For this review, take the finished solid that the model builds, in its own axes (mm). Round coordinates to 2 decimals unless told otherwise and drop trailing zeros. Write each loop counter-clockwise with the first axis right and the second up, starting at its lowest first coordinate (ties: lowest second). Pieces come first, ordered by that corner, then holes.
from build123d import *

# Parameters (mm, degrees)
BASE_DEPTH                     = 5.999988
MOUNTING_HOLES_D               = 4.4958
MOUNTING_HOLES_DEPTH           = 5.9944
SKETCH5_W                      = 6
SKETCH5_H                      = 12.7
F_4_BAR_MOUNT_DEPTH            = 131.351874194
SKETCH8_R                      = 2.2479
LIMIT_SWITCH_MOUNT_HOLES_DEPTH = 131.351874194
LIM_SW_CIRC_PATTERN_COUNT      = 2
SKETCH9_W                      = 25.4
SKETCH9_H                      = 63.5
SKETCH9_W_2                    = 47.975
WIRE_HOLES_DEPTH               = 131.351874194
FILLET1_R                      = 3.81


with BuildPart() as part:
    # Sketch1 → Base (new body)
    with BuildSketch(Plane(origin=(0, 0, 0), x_dir=(1, 0, 0), z_dir=(0, 1, 0))):
        Polygon((-38.138713756, 92.075), (-92.075, 38.138713756), (-92.075, -38.138713756), (-38.138713756, -92.075), (38.138713756, -92.075), (92.075, -38.138713756), (92.075, 38.138713756), (38.138713756, 92.075), align=None)
    extrude(amount=BASE_DEPTH)

    # Mounting holes
    with Locations(Plane(origin=(0, 5.999988, 0), x_dir=(1, 0, 0), z_dir=(0, 1, 0))):
        with Locations((-35.508457634, 85.725), (35.508457634, 85.725), (85.725, 35.508457634), (85.725, -35.508457634), (35.508457634, -85.725), (-35.508457634, -85.725), (-85.725, -35.508457634), (-85.725, 35.508457634)):
            Hole(MOUNTING_HOLES_D / 2, depth=MOUNTING_HOLES_DEPTH)

    # Sketch5 → 4-bar mount (cut, through all)
    with BuildSketch(Plane(origin=(0, 5.999988, 0), x_dir=(1, 0, 0), z_dir=(0, 1, 0))):
        with Locations((-22.05, 25.4)):
            Rectangle(SKETCH5_W, SKETCH5_H)
        with Locations((-22.05, -25.4)):
            Rectangle(SKETCH5_W, SKETCH5_H)
        with Locations((-22.05, 0)):
            Rectangle(SKETCH5_W, SKETCH5_H)
        with Locations((22.05, 0)):
            Rectangle(SKETCH5_W, SKETCH5_H)
        with Locations((22.05, -25.4)):
            Rectangle(SKETCH5_W, SKETCH5_H)
        with Locations((22.05, 25.4)):
            Rectangle(SKETCH5_W, SKETCH5_H)
    extrude(amount=-F_4_BAR_MOUNT_DEPTH, mode=Mode.SUBTRACT)

    # Sketch8 → limit switch mount holes (cut, through all)
    with BuildSketch(Plane(origin=(0, 5.999988, 0), x_dir=(1, 0, 0), z_dir=(0, 1, 0))):
        with Locations(Location((-35.508457634, 66.675, 0), (0, 0, 270))):
            Circle(SKETCH8_R)
        with Locations(Location((-23.67230509, 66.675, 0), (0, 0, 270))):
            Circle(SKETCH8_R)
        with Locations(Location((-11.836152545, 66.675, 0), (0, 0, 270))):
            Circle(SKETCH8_R)
        with Locations(Location((0, 66.675, 0), (0, 0, 270))):
            Circle(SKETCH8_R)
        with Locations(Location((11.836152545, 66.675, 0), (0, 0, 270))):
            Circle(SKETCH8_R)
        with Locations(Location((23.67230509, 66.675, 0), (0, 0, 270))):
            Circle(SKETCH8_R)
        with Locations(Location((35.508457634, 66.675, 0), (0, 0, 270))):
            Circle(SKETCH8_R)
    limit_switch_mount_holes = extrude(amount=-LIMIT_SWITCH_MOUNT_HOLES_DEPTH, mode=Mode.SUBTRACT)

    # lim sw circ pattern: limit switch mount holes ×2 about axis
    lim_sw_circ_pattern_axis = Axis((0, 0, 0), (0, 1, 0))
    for i in range(1, LIM_SW_CIRC_PATTERN_COUNT):
        add(limit_switch_mount_holes.rotate(lim_sw_circ_pattern_axis, i * 360 / LIM_SW_CIRC_PATTERN_COUNT), mode=Mode.SUBTRACT)

    # Sketch9 → Wire holes (cut, through all)
    with BuildSketch(Plane(origin=(0, 5.999988, 0), x_dir=(1, 0, 0), z_dir=(0, 1, 0))):
        Rectangle(SKETCH9_W, SKETCH9_H)
        with Locations((-55.3875, 0)):
            Rectangle(SKETCH9_W_2, SKETCH9_H)
        with Locations((55.3875, 0)):
            Rectangle(SKETCH9_W_2, SKETCH9_H)
        Polygon((-74.153201513, 38.1), (74.153201513, 38.1), (51.928201513, 60.325), (-51.928201513, 60.325), align=None)
        Polygon((-74.153201513, -38.1), (74.153201513, -38.1), (51.928201513, -60.325), (-51.928201513, -60.325), align=None)
    extrude(amount=-WIRE_HOLES_DEPTH, mode=Mode.SUBTRACT)

    # Fillet1
    fillet1_edges = [part.edges().sort_by_distance(p)[0] for p in [
        (-12.7, 2.999994, 31.75),
        (-12.7, 2.999994, -31.75),
        (12.7, 2.999994, -31.75),
        (12.7, 2.999994, 31.75),
        (-79.375, 2.999994, 31.75),
        (-79.375, 2.999994, -31.75),
        (-31.4, 2.999994, -31.75),
        (-31.4, 2.999994, 31.75),
        (31.4, 2.999994, 31.75),
        (31.4, 2.999994, -31.75),
        (79.375, 2.999994, -31.75),
        (79.375, 2.999994, 31.75),
        (-74.153201513, 2.999994, -38.1),
        (-51.928201513, 2.999994, -60.325),
        (51.928201513, 2.999994, -60.325),
        (74.153201513, 2.999994, -38.1),
        (-51.928201513, 2.999994, 60.325),
        (-74.153201513, 2.999994, 38.1),
        (74.153201513, 2.999994, 38.1),
        (51.928201513, 2.999994, 60.325),
    ]]
    fillet(fillet1_edges, radius=FILLET1_R)


solid = part.part
(1) We need section B-B, the plane x = 0. Give the boundary of the cut face in (y, z) (3 decimals), and give its area (3 significant figures).
Geometry check:
outline: (0, -92.075) - (6, -92.075) - (6, -68.923) - (0, -68.923) - close; (0, -64.427) - (6, -64.427) - (6, -60.325) - (0, -60.325) - close; (0, -38.1) - (6, -38.1) - (6, -31.75) - (0, -31.75) - close; (0, 31.75) - (6, 31.75) - (6, 38.1) - (0, 38.1) - close; (0, 60.325) - (6, 60.325) - (6, 64.427) - (0, 64.427) - close; (0, 68.923) - (6, 68.923) - (6, 92.075) - (0, 92.075) - close
area: 403 mm2
(2) We need section C-C, the plane z = -52.5. Give the boundary of the cut face in (x, y).
Geometry check:
outline: (-77.71, 0) - (-59.75, 0) - (-59.75, 6) - (-77.71, 6) - close; (59.75, 0) - (77.71, 0) - (77.71, 6) - (59.75, 6) - close
(3) We need section D-D, the plane x = 73. Give the boundary of the cut face in (y, z), and give its area (3 significant figures).
Geometry check:
outline: (0, -57.21) - (6, -57.21) - (6, -31.75) - (0, -31.75) - close; (0, 31.75) - (6, 31.75) - (6, 57.21) - (0, 57.21) - close
area: 306 mm2
(4) We need section A-A, the plane z = 14.5. Give the boundary of the cut face in (x, y) (3 decimals).
Geometry check:
outline: (-92.075, 0) - (-79.375, 0) - (-79.375, 6) - (-92.075, 6) - close; (-31.4, 0) - (-12.7, 0) - (-12.7, 6) - (-31.4, 6) - close; (12.7, 0) - (31.4, 0) - (31.4, 6) - (12.7, 6) - close; (79.375, 0) - (92.075, 0) - (92.075, 6) - (79.375, 6) - close
(5) Mouldability with a two-part tool opening along Z and no side actions: class faces 1 (the face through (87.97, 2.96, -35.61)), 2 (the face through (-1, 3, 92.075)) as pulls with the +Z half, pulls with the -Z half, needs draft (parallel to the pull), parting line crosses it, or undercut.
Geometry check:
face 1: undercut
face 2: pulls with the +Z half
(6) For line 1 along X through (y, z) = (0.25, -13) (3 decimals); line 2 along X through (y, z) = (4.3, -23) (3 decimals); line 3 along Z through (x, y) = (26, 3.05) (3 decimals), list the stretches that pass through material, from the lowest coordinate up.
Geometry check:
line 1: x = -92.075 to -79.375, -31.4 to -12.7, 12.7 to 31.4, 79.375 to 92.075
line 2: x = -92.075 to -79.375, -31.4 to -25.05, -19.05 to -12.7, 12.7 to 19.05, 25.05 to 31.4, 79.375 to 92.075
line 3: z = -92.075 to -60.325, -38.1 to 38.1, 60.325 to 92.075
(7) For pin 1 Ø2 at (y, z) = (4, 55) entering from +X; pin 2 Ø3.5 at (x, z) = (-23.67, 66.68) entering from +Y; pin 3 Ø1 at (x, y) = (-44.5, 3) entering from +Z; pin 4 Ø2 at (x, z) = (34.5, 85.5) entering from +Y, all flat-tipped, find the tip position at first contact; note any pin that passes through.
Geometry check:
pin 1: stops at x = 76.21
pin 2: passes through
pin 3: stops at z = 86.21
pin 4: stops at y = 0.01
